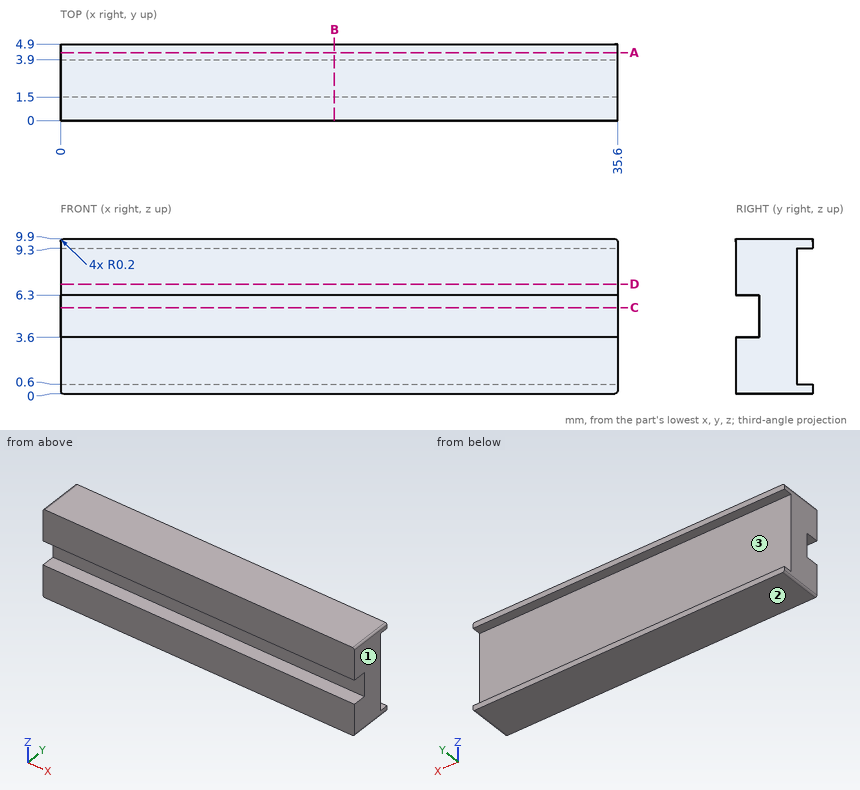
Part print with two shaded views. Sizes in mm from the minimum x, y, z corner. Round coordinates to 2 decimals unless told otherwise and drop trailing zeros. Loops run counter-clockwise (first coordinate to the right, second up) from the corner with the lowest first, then second, coordinate; pieces in that order, holes last. Notation, with made-up numbers: (57, 88.25) - (81, 88.25) arc R11 cw to (81, 100.25) - close; hole circle Ø6 at (81.5, 38). An arc over 180 degrees is marked (long way). Answer as a JSON object with one key per item and string values.
Item 1: Pin check, flat tips, straight feed: pin 1 (0.8 mm diameter, centred on x = 21, z = 5.5, fed in from -Y); pin 2 (1 mm diameter, centred on x = 14, z = 6.5, fed in from +Y). Stop position of each tip, or through.
Output:
{"pin 1": "y = 1.5", "pin 2": "y = 3.9"}
Item 2: Wall check: L1, parallel to Z at x = 23.5, y = 1.1; L2, parallel to Z at x = 24.5, y = 4.15; L3, parallel to Y at x = 8.5, z = 1. Give the ranges that are in metal, low to high.
Output:
{"L1": "0 to 3.6, 6.3 to 9.9", "L2": "0 to 0.6, 9.3 to 9.9", "L3": "0 to 3.9"}
Item 3: Band-saw the part on D-D on z = 7. List the corners of the cut face in (x, y), plus the area to 3 significant figures.
Output:
{"outline": "(0, 0) - (35.6, 0) - (35.6, 3.9) - (0, 3.9) - close", "area": "139 mm2"}
Item 4: Pull direction Z, two halves, no side cores. Call the marked faces 1, 2 and 3: pulls with the +Z half, pulls with the -Z half, needs draft (parallel to the pull), parting line crosses it, or undercut.
Output:
{"face 1": "needs draft", "face 2": "pulls with the -Z half", "face 3": "undercut"}
Item 5: Band-saw the part on B-B on x = 17.5. List the corners of the cut face in (y, z).
Output:
{"outline": "(0, 0) - (4.9, 0) - (4.9, 0.6) - (3.9, 0.6) - (3.9, 9.3) - (4.9, 9.3) - (4.9, 9.9) - (0, 9.9) - (0, 6.3) - (1.5, 6.3) - (1.5, 3.6) - (0, 3.6) - close"}
Item 6: Band-saw the part on C-C on z = 5.5. List the corners of the cut face in (x, y).
Output:
{"outline": "(0, 1.5) - (35.6, 1.5) - (35.6, 3.9) - (0, 3.9) - close"}
Item 7: Band-saw the part on A-A on y = 4.35. List the corners of the cut face in (x, z).
Output:
{"outline": "(0, 0.2) arc R0.2 ccw to (0.2, 0) - (35.4, 0) arc R0.2 ccw to (35.6, 0.2) - (35.6, 0.6) - (0, 0.6) - close; (0, 9.3) - (35.6, 9.3) - (35.6, 9.7) arc R0.2 ccw to (35.4, 9.9) - (0.2, 9.9) arc R0.2 ccw to (0, 9.7) - close"}
